```python
from build123d import *

# Parameters (mm, degrees)
SKETCH1_W                      = 32
SKETCH1_H                      = 32
SKETCH1_R                      = 7.5
BOSS_EXTRUDE1_DEPTH            = 20
CBORE_FOR_M3_SHCS1_D           = 3.4
CBORE_FOR_M3_SHCS1_CBORE_D     = 6.5
CBORE_FOR_M3_SHCS1_CBORE_DEPTH = 3
M5X0_8_TAPPED_HOLE1_REACH      = 42.988
M5X0_8_TAPPED_HOLE1_BORE_R     = 2.1
CHAMFER1_SIZE                  = 3


with BuildPart() as part:
    # Sketch1 → Boss-Extrude1 (new body)
    with BuildSketch(Plane(origin=(0, 0, 0), x_dir=(1, 0, 0), z_dir=(0, 1, 0))):
        Rectangle(SKETCH1_W, SKETCH1_H)
        with Locations(Location((0, 0, 0), (0, 0, 270))):
            Circle(SKETCH1_R, mode=Mode.SUBTRACT)
    extrude(amount=BOSS_EXTRUDE1_DEPTH)

    # CBORE for M3 SHCS1 (through all)
    with Locations(Plane(origin=(0, 0, 0), x_dir=(-1, 0, 0), z_dir=(0, -1, 0))):
        with Locations((-11, -11), (11, -11), (11, 11), (-11, 11)):
            CounterBoreHole(CBORE_FOR_M3_SHCS1_D / 2, CBORE_FOR_M3_SHCS1_CBORE_D / 2, CBORE_FOR_M3_SHCS1_CBORE_DEPTH)

    # M5x0.8 Tapped Hole1 bore → M5x0.8 Tapped Hole1 (cut, up to next)
    with BuildSketch(Plane.XY.offset(16), mode=Mode.PRIVATE) as m5x0_8_tapped_hole1_sk1:
        with Locations((0, 8)):
            Circle(M5X0_8_TAPPED_HOLE1_BORE_R)
    m5x0_8_tapped_hole1_tool1 = extrude(m5x0_8_tapped_hole1_sk1.sketch, amount=-M5X0_8_TAPPED_HOLE1_REACH, mode=Mode.PRIVATE) & part.part
    add(m5x0_8_tapped_hole1_tool1.solids().sort_by_distance((0, 8, 16))[0], mode=Mode.SUBTRACT)

    # Chamfer1
    chamfer1_edges = [part.edges().sort_by_distance(p)[0] for p in [
        (16, 10, 16),
        (-16, 10, 16),
        (-16, 10, -16),
        (16, 10, -16),
    ]]
    chamfer(chamfer1_edges, length=CHAMFER1_SIZE)


solid = part.part
```
Check sheet for the modelled part. Datum: model origin and axes. Units: mm. A direction names the side the tool comes from. Round coordinates to 2 decimals unless told otherwise and drop trailing zeros. Write each loop counter-clockwise with the first axis right and the second up, starting at its lowest first coordinate (ties: lowest second). Pieces come first, ordered by that corner, then holes. Notation, with made-up numbers: M -9.75,31.5 L 11.25,31.5 A28 cw 11.25,62.5 Z; hole C 17.25,-22 d2. An arc over 180 degrees is marked long. Write item = value, one per line. Start each with the question number.
1. Gauge pin test, flat ends, axial feed: pin 1 (2.5 mm diameter, centred on x = 11, z = 11, fed in from -Y); pin 2 (4 mm diameter, centred on x = 11, z = -11, fed in from -Y); pin 3 (2.5 mm diameter, centred on x = 0, y = 8, fed in from +Z). Record the tip position at first contact, or that the pin passes through.
2. Tool access check on faces 1 (the flat face through (-16, 10, 0)), 2 (the cylindrical face through (13.395, 1.479, 8.803)). Record the directions out of +Z, -Z, +X, -X, +Y, -Y that give a thin tool (end or side, any length) a straight path to the whole face; none if there is none.
3. Scan lines: line 1 (X direction, y = 10, z = -11); line 2 (X direction, y = 1.85, z = 11). Record each from-to range of solid material in increasing order. Write a range as [from, to].
4. Release check for a two-part mould opening along Y. For faces 3 (the flat face through (7, 20, -4)), 4 (the cylindrical face through (-0.273, 10.082, 11.661)), 5 (the cylindrical face through (14.247, 1.479, -11.143)) record: pulls with the +Y half, pulls with the -Y half, needs draft (parallel to the pull), parting line crosses it, or undercut.
5. Section check C-C, the plane z = 11. Record the cut outline in (x, y), then the cut area to 3 significant figures.
6. Section check A-A, the plane x = 11. Record the cut outline in (y, z), then the cut area to 3 significant figures.
7. Section check B-B, the plane z = -11. Record the cut outline in (x, y).
8. Section check D-D, the plane y = 8. Record the cut outline in (x, z), then the cut area to 3 significant figures.
Results found:
q1.pin_1 = through
q1.pin_2 = 3
q1.pin_3 = -7.4
q2.face_1 = +Z, -Z, -X, +Y, -Y
q2.face_2 = -Y
q3.line_1 = [-16, -12.7], [-9.3, 9.3], [12.7, 16]
q3.line_2 = [-16, -14.25], [-7.75, 7.75], [14.25, 16]
q4.face_3 = pulls with the +Y half
q4.face_4 = undercut
q4.face_5 = needs draft
q5.outline = M -16,0 L -14.25,0 L -14.25,3 L -12.7,3 L -12.7,20 L -16,20 Z; M -9.3,3 L -7.75,3 L -7.75,0 L 7.75,0 L 7.75,3 L 9.3,3 L 9.3,20 L -9.3,20 Z; M 12.7,3 L 14.25,3 L 14.25,0 L 16,0 L 16,20 L 12.7,20 Z; hole C 0,8 d4.2
q5.area = 472 mm^2
q6.outline = M 0,-16 L 20,-16 L 20,-12.7 L 3,-12.7 L 3,-14.25 L 0,-14.25 Z; M 0,-7.75 L 3,-7.75 L 3,-9.3 L 20,-9.3 L 20,9.3 L 3,9.3 L 3,7.75 L 0,7.75 Z; M 0,14.25 L 3,14.25 L 3,12.7 L 20,12.7 L 20,16 L 0,16 Z
q6.area = 485 mm^2
q7.outline = M -16,0 L -14.25,0 L -14.25,3 L -12.7,3 L -12.7,20 L -16,20 Z; M -9.3,3 L -7.75,3 L -7.75,0 L 7.75,0 L 7.75,3 L 9.3,3 L 9.3,20 L -9.3,20 Z; M 12.7,3 L 14.25,3 L 14.25,0 L 16,0 L 16,20 L 12.7,20 Z
q8.outline = M -16,-13 L -13,-16 L 13,-16 L 16,-13 L 16,13 L 13,16 L 2.1,16 L 2.1,7.2 A7.5 cw long -2.1,7.2 L -2.1,16 L -13,16 L -16,13 Z; hole C -11,-11 d3.4; hole C -11,11 d3.4; hole C 11,-11 d3.4; hole C 11,11 d3.4
q8.area = 757 mm^2
